Could you check a few things on this drawing? It's one solid part, dimensions in mm from its lowest x, y, z. A direction names the side the tool comes from. Coordinates: 2 decimals unless noted, no trailing zeros. Loops run counter-clockwise (first coordinate to the right, second up) from the corner with the lowest first, then second, coordinate; pieces in that order, holes last.
1) Imagine slicing it at C-C on y = 2.25. Please give me the cut outline in (x, z).
2) Imagine slicing it at D-D on z = 82.5. Please give me the cut outline in (x, y).
3) Imagine slicing it at A-A on z = 57. Please give me the cut outline in (x, y) (1 decimal).
4) Will these pins go through, and if not, where does the flat tip stop? P1, Ø4, axis at y = 6, z = 36, coming from the +X side; P2, Ø6, axis at x = 18, z = 9.5, coming from the +Y side; P3, Ø10, axis at x = 25, y = 5, coming from the +Z side.
5) Thinking about a two-plate mould opening in X: for the marked faces 1, 2 and 3, which applies, released by +X, released by -X, zero draft, split by the parting line, or undercut?
6) If I drill on line 1 along X through (y, z) = (2.5, 55.5); line 2 along Y through (x, z) = (84.5, 51); line 3 along X through (y, z) = (14, 64.5), over which ranges is the centre line in solid material (lowest first)?
7) For the marked faces 4, 5 and 6, which set-ups out of +Z, -Z, +X, -X, +Y, -Y let a thin tool reach every point of the face, with its end or its side?
8) Imagine slicing it at B-B on x = 44.5. Please give me the cut outline in (y, z), plus the area to 3 significant figures.
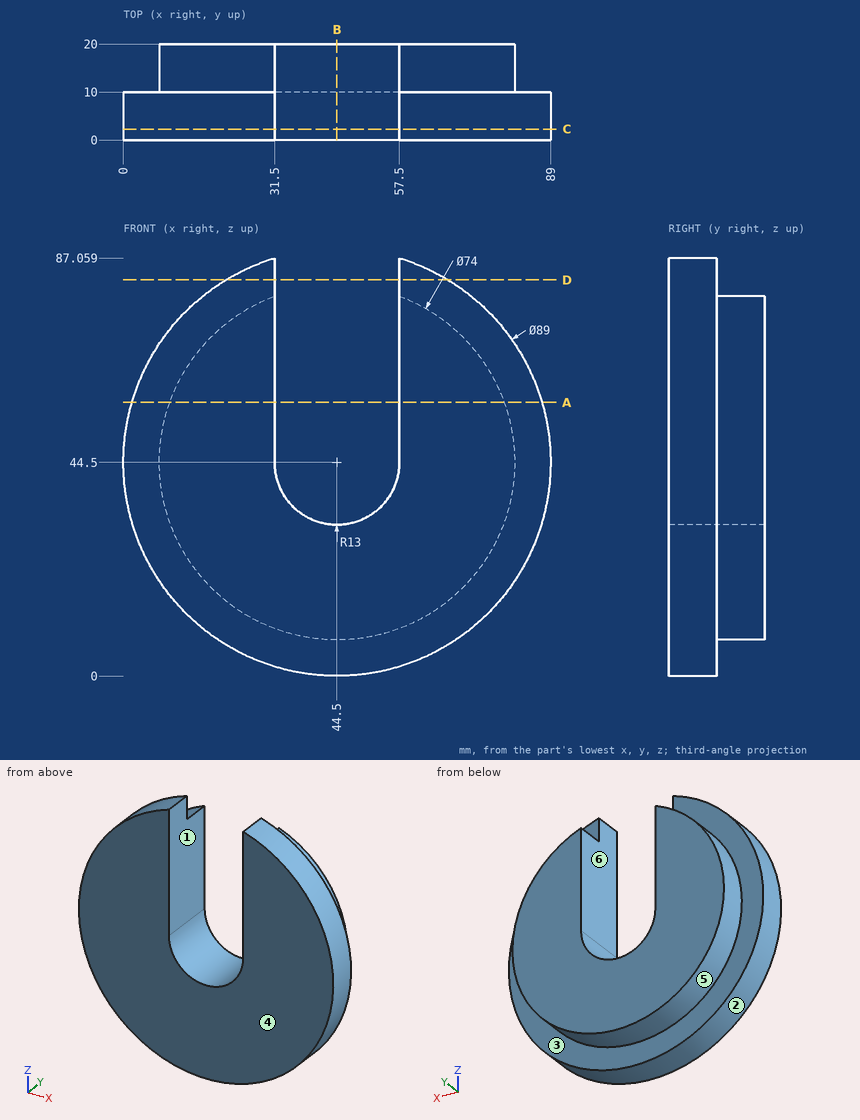
Filled in:
1. outline: (31.5, 44.5) - (31.5, 87.06) arc R44.5 ccw (long way) to (57.5, 87.06) - (57.5, 44.5) arc R13 cw to start
2. outline: (21.34, 0) - (31.5, 0) - (31.5, 10) - (21.34, 10) - close; (57.5, 0) - (67.66, 0) - (67.66, 10) - (57.5, 10) - close
3. outline: (1.8, 0) - (31.5, 0) - (31.5, 20) - (9.7, 20) - (9.7, 10) - (1.8, 10) - close; (57.5, 0) - (87.2, 0) - (87.2, 10) - (79.3, 10) - (79.3, 20) - (57.5, 20) - close
4. P1: stops at x = 88.52
4. P2: stops at y = 10
4. P3: stops at z = 86.57
5. face 1: undercut
5. face 2: split by the parting line
5. face 3: zero draft
6. line 1: x = 1.38 to 31.5, 57.5 to 87.62
6. line 2: y = 0 to 10
6. line 3: x = 13.37 to 31.5, 57.5 to 75.63
7. face 4: +Z, -Z, +X, -X, -Y
7. face 5: +Y
7. face 6: +Z, +Y, -Y
8. outline: (0, 0) - (10, 0) - (10, 7.5) - (20, 7.5) - (20, 31.5) - (0, 31.5) - close
8. area: 555 mm2
